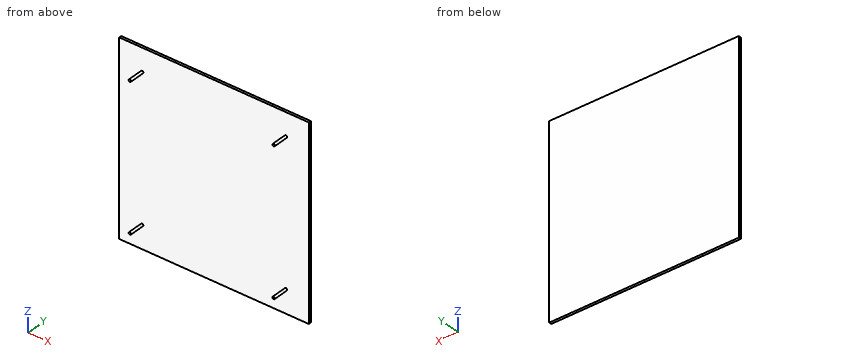
```python
from build123d import *

# Parameters (mm, degrees)
SKETCH_1_W      = 310
SKETCH_1_H      = 310
EXTRUDE_1_DEPTH = 4
SKETCH_2_R      = 2
EXTRUDE_2_DEPTH = 25


with BuildPart() as part:
    # Эскиз1 → Бобышка-Вытянуть1 (new body)
    with BuildSketch(Plane(origin=(0, 0, 0), x_dir=(1, 0, 0), z_dir=(0, 1, 0))):
        with Locations((155, 155)):
            Rectangle(SKETCH_1_W, SKETCH_1_H)
    extrude(amount=EXTRUDE_1_DEPTH)

    # Эскиз2 → Бобышка-Вытянуть2 (add)
    with BuildSketch(Plane.XZ):
        with Locations(Location((272.5, -37.5, 0), (0, 0, 270))):
            Circle(SKETCH_2_R)
        with Locations(Location((272.5, -272.5, 0), (0, 0, 270))):
            Circle(SKETCH_2_R)
        with Locations(Location((37.5, -37.5, 0), (0, 0, 270))):
            Circle(SKETCH_2_R)
        with Locations(Location((37.5, -272.5, 0), (0, 0, 270))):
            Circle(SKETCH_2_R)
    extrude(amount=EXTRUDE_2_DEPTH)


solid = part.part
```
Design review of the part built by this model. Coordinates are the model's own, in mm. Round coordinates to 2 decimals unless told otherwise and drop trailing zeros. Order: outer loops, then holes, each group sorted by start corner. A loop starts at its lowest first (then second) coordinate and runs counter-clockwise, first axis right, second up. Notation, with made-up numbers: (84, 64.25) - (141, 64.25) arc R9 cw to (141, 80.25) - close; hole circle Ø6 at (26.25, 55.25). An arc over 180 degrees is marked (long way). Return JSON: item names as keys, results as strings.
Q1. Wall thickness on L1, parallel to X at y = -9, z = -38; L2, parallel to Y at x = 285, z = -77.5; L3, parallel to X at y = -9.75, z = -274: over which ranges is each line inside the solid? List them lowest first. Write a range as [from, to].
Computed values:
{"L1": "x = [35.56, 39.44], [270.56, 274.44]", "L2": "y = [0, 4]", "L3": "x = [36.18, 38.82], [271.18, 273.82]"}
Q2. For pin 1 Ø10 at (y, z) = (-14, -38.5) entering from -X; pin 2 Ø10 at (x, z) = (36, -174.5) entering from -Y; pin 3 Ø8 at (y, z) = (-4.5, -277) entering from +X, all flat-tipped, find the tip position at first contact; note any pin that passes through.
Computed values:
{"pin 1": "stops at x = 35.5", "pin 2": "stops at y = 0", "pin 3": "stops at x = 274.44"}
Q3. Consider section B-B on x = 137.5. Write out the cut boundary in (y, z).
Computed values:
{"outline": "(0, -310) - (4, -310) - (4, 0) - (0, 0) - close"}
Q4. Consider section A-A on y = -19.5. Write out the cut boundary in (x, z), plus the area to 3 significant figures.
Computed values:
{"outline": "circle Ø4 at (37.5, -272.5); circle Ø4 at (37.5, -37.5); circle Ø4 at (272.5, -272.5); circle Ø4 at (272.5, -37.5)", "area": "50.3 mm2"}
Q5. Consider section C-C on z = -222. Write out the cut boundary in (x, y).
Computed values:
{"outline": "(0, 0) - (310, 0) - (310, 4) - (0, 4) - close"}
